from build123d import *

# Parameters (mm, degrees)
BOSS_EXTRUDE1_DEPTH = 30
FILLET1_R           = 10
SKETCH2_R           = 2.5
CUT_EXTRUDE1_DEPTH  = 30.15
SKETCH3_R           = 4.5
CUT_EXTRUDE2_DEPTH  = 20


with BuildPart() as part:
    # Sketch1 → Boss-Extrude1 (new body)
    with BuildSketch(Plane.XY):
        with BuildLine():
            Line((-26.797076023, 29.15), (-35.15, 0))
            Line((-35.15, 0), (-19.15, 0))
            ThreePointArc((-19.15, 0), (0, 19.15), (19.15, 0))
            Line((19.15, 0), (35.15, 0))
            Line((35.15, 0), (26.797076023, 29.15))
            Line((26.797076023, 29.15), (-26.797076023, 29.15))
        make_face()
    extrude(amount=BOSS_EXTRUDE1_DEPTH)

    # Fillet1
    fillet1_edges = [part.edges().sort_by_distance(p)[0] for p in [
        (-26.797076023, 29.15, 15),
        (26.797076023, 29.15, 15),
    ]]
    fillet(fillet1_edges, radius=FILLET1_R)

    # Sketch2 → Cut-Extrude1 (cut, through all)
    with BuildSketch(Plane.XZ):
        with Locations((-27.15, 15)):
            Circle(SKETCH2_R)
        with Locations((27.15, 15)):
            Circle(SKETCH2_R)
    extrude(amount=-CUT_EXTRUDE1_DEPTH, mode=Mode.SUBTRACT)

    # Sketch3 → Cut-Extrude2 (cut)
    with BuildSketch(Plane(origin=(0, 29.15, 0), x_dir=(1, 0, 0), z_dir=(0, 1, 0))):
        with Locations((27.15, -15)):
            Circle(SKETCH3_R)
        with Locations((-27.15, -15)):
            Circle(SKETCH3_R)
    extrude(amount=-CUT_EXTRUDE2_DEPTH, mode=Mode.SUBTRACT)


solid = part.part
CAD build for the part. Positions are in the model's coordinates, mm. A direction names the side the tool comes from. Coordinates: 2 decimals unless noted, no trailing zeros. Order: outer loops, then holes, each group sorted by start corner. A loop starts at its lowest first (then second) coordinate and runs counter-clockwise, first axis right, second up.
Item 1: Band-saw the part on A-A on y = 5.75. List the corners of the cut face in (x, z).
Check sheet entries:
outline: (-33.5, 0) - (-18.27, 0) - (-18.27, 30) - (-33.5, 30) - close; (18.27, 0) - (33.5, 0) - (33.5, 30) - (18.27, 30) - close; hole circle Ø5 at (-27.15, 15); hole circle Ø5 at (27.15, 15)
Item 2: Drill centre lines: L1, parallel to Z at x = -27.15, y = 2.75; L2, parallel to Z at x = -27.15, y = 20.5; L3, parallel to X at y = 14.75, z = 11.5. Where is each one in solid material? Low to high.
Check sheet entries:
L1: z = 0 to 12.5, 17.5 to 30
L2: z = 0 to 10.5, 19.5 to 30
L3: x = -30.92 to -29.98, -24.32 to -12.21, 12.21 to 24.32, 29.98 to 30.92
Item 3: Band-saw the part on D-D on z = 15. List the corners of the cut face in (x, y).
Check sheet entries:
outline: (-35.15, 0) - (-29.65, 0) - (-29.65, 9.15) - (-31.65, 9.15) - (-31.65, 12.21) - close; (-24.65, 0) - (-19.15, 0) arc R19.15 cw to (19.15, 0) - (24.65, 0) - (24.65, 9.15) - (22.65, 9.15) - (22.65, 28.56) arc R10 ccw to (19.26, 29.15) - (-19.26, 29.15) arc R10 ccw to (-22.65, 28.56) - (-22.65, 9.15) - (-24.65, 9.15) - close; (29.65, 0) - (35.15, 0) - (31.65, 12.21) - (31.65, 9.15) - (29.65, 9.15) - close
Item 4: Two-plate mould, pull along Z, no slides. Class faces 1 (the face through (29.46, 4.51, 14.04)), 2 (the face through (32, 11, 15)), 3 (the face through (0, 21, 30)): +Z half, -Z half, draft (parallel to the pull), parting line (faces both ways), or undercut.
Check sheet entries:
face 1: undercut
face 2: draft
face 3: +Z half
Item 5: Band-saw the part on B-B on y = 16. List the corners of the cut face in (x, z), plus the area to 3 significant figures.
Check sheet entries:
outline: (-30.57, 0) - (-10.52, 0) - (-10.52, 30) - (-30.57, 30) - (-30.57, 17.93) arc R4.5 cw (long way) to (-30.57, 12.07) - close; (10.52, 0) - (30.57, 0) - (30.57, 12.07) arc R4.5 cw (long way) to (30.57, 17.93) - (30.57, 30) - (10.52, 30) - close
area: 1,080 mm2
Item 6: Band-saw the part on C-C on x = -27.15. List the corners of the cut face in (y, z).
Check sheet entries:
outline: (0, 0) - (25.29, 0) - (25.29, 10.5) - (9.15, 10.5) - (9.15, 12.5) - (0, 12.5) - close; (0, 17.5) - (9.15, 17.5) - (9.15, 19.5) - (25.29, 19.5) - (25.29, 30) - (0, 30) - close
Item 7: Pin check, flat tips, straight feed: pin 1 Ø2.5 at (x, z) = (-29, 17) entering from +Y; pin 2 Ø1.5 at (y, z) = (22.5, 10) entering from +X; pin 3 Ø5 at (y, z) = (19.5, 6) entering from -X. Stop position of each tip, or through.
Check sheet entries:
pin 1: stops at y = 9.15
pin 2: stops at x = 28.92
pin 3: stops at x = -30.28
Item 8: 3-axis set-ups, long thin cutter, end or side, ignore diameter. For faces 4 (the face through (-22.858, 16.833, 13.648)), 5 (the face through (-27, 0, 11)): which of +Z, -Z, +X, -X, +Y, -Y reach the whole face in a straight line?
Check sheet entries:
face 4: +Y
face 5: +Z, -Z, +X, -X, -Y
